Can you work these out from the model? Positions are in its coordinate system, mm. Face numbers are marked on the shaded views. A direction names the side the tool comes from. Give positions to 0.01 mm unless a question says otherwise; leave off trailing zeros. Loops run counter-clockwise (first coordinate to the right, second up) from the corner with the lowest first, then second, coordinate; pieces in that order, holes last. Notation, with made-up numbers: (-33.75, -35.5) -> (-26.75, -35.5) arc R29 cw to (-26.75, 0.5) -> close; hole circle Ø1 at (15, 79). An arc over 180 degrees is marked (long way). One line per question, with ' | ' between items.
from build123d import *

# Parameters (mm, degrees)
F1_DEPTH             = 12.7
F4_D                 = 3.175
F4_DEPTH             = 25.4
F4_CSINK_D           = 9.1186
F4_CSINK_ANGLE       = 82
F4_TIP               = 0.9538662327
F4_ON_F2_D           = 3.175
F4_ON_F2_DEPTH       = 25.4
F4_ON_F2_CSINK_D     = 9.1186
F4_ON_F2_CSINK_ANGLE = 82
F4_ON_F2_TIP         = 0.9538662327


with BuildPart() as f1:
    # F0 (on Front) → F1 (new body, symmetric)
    with BuildSketch(Plane.XZ):
        with BuildLine():
            Line((-3.175, -30.48), (-25.4, -30.48))
            Line((-25.4, -30.48), (-25.4, -32.305))
            ThreePointArc((-25.4, -32.305), (-24.4700640303, -34.5500640303), (-22.225, -35.48))
            Line((-22.225, -35.48), (3.175, -35.48))
            ThreePointArc((3.175, -35.48), (5.4200640303, -34.5500640303), (6.35, -32.305))
            Line((6.35, -32.305), (6.35, 8.97))
            ThreePointArc((6.35, 8.97), (8.2098719395, 13.4601280605), (12.7, 15.32))
            Line((12.7, 15.32), (34.925, 15.32))
            ThreePointArc((34.925, 15.32), (37.1700640303, 16.2499359697), (38.1, 18.495))
            Line((38.1, 18.495), (38.1, 20.32))
            Line((38.1, 20.32), (-22.225, 20.32))
            ThreePointArc((-22.225, 20.32), (-24.4700640303, 19.3900640303), (-25.4, 17.145))
            Line((-25.4, 17.145), (-25.4, 3.175))
            ThreePointArc((-25.4, 3.175), (-24.4700640303, 0.9299359697), (-22.225, 0))
            Line((-22.225, 0), (-3.175, 0))
            ThreePointArc((-3.175, 0), (-0.9299359697, -0.9299359697), (0, -3.175))
            Line((0, -3.175), (0, -27.305))
            ThreePointArc((0, -27.305), (-0.9299359697, -29.5500640303), (-3.175, -30.48))
        make_face()
    extrude(amount=F1_DEPTH, both=True)

    # F4
    with Locations(Plane(origin=(0, 0, 15.32), x_dir=(1, 0, 0), z_dir=(0, 0, -1))):
        with Locations((23.8125, 0)):
            CounterSinkHole(F4_D / 2, F4_CSINK_D / 2, depth=F4_DEPTH, counter_sink_angle=F4_CSINK_ANGLE)
            with Locations((0, 0, -(F4_DEPTH + F4_TIP / 2))):  # 118° drill point
                Cone(0, F4_D / 2, F4_TIP, mode=Mode.SUBTRACT)

    # F4 on F2
    with Locations(Plane(origin=(0, 0, -35.48), x_dir=(1, 0, 0), z_dir=(0, 0, -1))):
        with Locations((-9.525, 0)):
            CounterSinkHole(F4_ON_F2_D / 2, F4_ON_F2_CSINK_D / 2, depth=F4_ON_F2_DEPTH, counter_sink_angle=F4_ON_F2_CSINK_ANGLE)
            with Locations((0, 0, -(F4_ON_F2_DEPTH + F4_ON_F2_TIP / 2))):  # 118° drill point
                Cone(0, F4_ON_F2_D / 2, F4_ON_F2_TIP, mode=Mode.SUBTRACT)


solid = f1.part
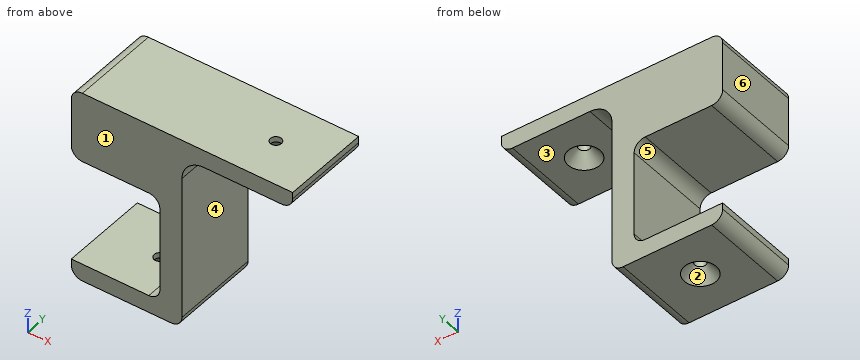
Q1. If we section it at C-C (z = 5.5): Write out the boundary of the cut face in (x, y), plus the area to 3 significant figures.
Entries:
outline: (-25.4, -12.7) -> (6.35, -12.7) -> (6.35, 12.7) -> (-25.4, 12.7) -> close | area: 806 mm²
Q2. If we mould it in two halves opening along Y, with no side actions, what happens to the marked faces 1, 2 and 3? For each: pulls with the +Y half, pulls with the -Y half, needs draft (parallel to the pull), parting line crosses it, or undercut.
Entries:
face 1: pulls with the -Y half | face 2: undercut | face 3: needs draft
Q3. If we section it at A-A (y = 0): State how many separate pieces and enclosed holes the cut face has, plus the area to 3 significant figures.
Entries:
separate pieces: 3 | enclosed holes: 0 | area: 1,110 mm²
Q4. If I drill on probe 1 along Z at (x, y) = (-19, 10.75); probe 2 along Z at (x, y) = (12.5, 3.5); probe 3 along X at (y, z) = (-3.75, -32), over which ranges is the centre line in solid material (lowest first)? Write a range as from..to.
Entries:
probe 1: -35.48..-30.48, 0..20.32 | probe 2: 15.32..20.32 | probe 3: -25.4..6.35
Q5. If we section it at B-B (y = -10.25): Write out the boundary of the cut face in (x, z) (3 decimals).
Entries:
outline: (-25.4, -32.305) arc R3.175 ccw to (-22.225, -35.48) -> (3.175, -35.48) arc R3.175 ccw to (6.35, -32.305) -> (6.35, 8.97) arc R6.35 cw to (12.7, 15.32) -> (34.925, 15.32) arc R3.175 ccw to (38.1, 18.495) -> (38.1, 20.32) -> (-22.225, 20.32) arc R3.175 ccw to (-25.4, 17.145) -> (-25.4, 3.175) arc R3.175 ccw to (-22.225, 0) -> (-3.175, 0) arc R3.175 cw to (0, -3.175) -> (0, -27.305) arc R3.175 cw to (-3.175, -30.48) -> (-25.4, -30.48) -> close
Q6. On a 3-axis mill with a long thin cutter (end or side, diameter ignored), from which of +Z, -Z, +X, -X, +Y, -Y can I reach the whole of each face in a straight line? I mean the marked faces 4, 5 and 6. Say none if no direction works.
Entries:
face 4: -Z, +X, +Y, -Y | face 5: -X, +Y, -Y | face 6: +Z, -Z, -X, +Y, -Y
Q7. For pin 1 Ø6 at (x, z) = (9.5, -22.5) entering from +Y; pin 2 Ø4 at (x, y) = (-9.525, 0) entering from -Z; pin 3 Ø12 at (y, z) = (5.5, -15) entering from -X, each with a flat end and sliding along its axis, tell me the tip position at first contact or that it passes through.
Entries:
pin 1: through | pin 2: z = -32.54 | pin 3: x = 0
Q8. If we section it at D-D (z = -6): Write out the boundary of the cut face in (x, y), plus the area to 3 significant figures.
Entries:
outline: (0, -12.7) -> (6.35, -12.7) -> (6.35, 12.7) -> (0, 12.7) -> close | area: 161 mm²
